Read the model definition and answer for the solid it produces. Units are mm, in the model's axes. A direction names the side the tool comes from. Round coordinates to 2 decimals unless told otherwise and drop trailing zeros. Write each loop counter-clockwise with the first axis right and the second up, starting at its lowest first coordinate (ties: lowest second). Pieces come first, ordered by that corner, then holes. Notation, with made-up numbers: (-9, 89) - (21, 89) arc R20 cw to (21, 111) - close; hole circle Ø9 at (-25.5, 72.25). An arc over 180 degrees is marked (long way). Answer as CSV lines item,"result". Start each with the question number.
1) Each of these flat-tipped pins is pushed along its axis until it touches: pin 1 (8 mm diameter, centred on x = 15.5, y = 5, fed in from +Z); pin 2 (8 mm diameter, centred on y = 12.5, z = 2.5, fed in from +X). Where does it stop, or does it pass through?
2) Find section D-D on z = 4.5. Determine the outline of the cut face in (x, y).
3) Find section A-A on x = 21.25. Determine the outline of the cut face in (y, z).
4) For a pull along Y with two mould halves and no side action, classify faces 3 (the flat face through (10, 0, 13)), 4 (the flat face through (10, 25.4, 13)), 5 (the flat face through (11, 23.812, 15)), 6 (the flat face through (1, 13, 0)) as +Y half, -Y half, draft (parallel to the pull), parting line (faces both ways), or undercut.
5) Find section C-C on y = 2.75. Determine the outline of the cut face in (x, z), then the cut area to 3 significant figures.
6) Which of the six approach directions +Z, -Z, +X, -X, +Y, -Y give full straight-line access (tool end or side, diameter ignored) to faces 1 (the flat face through (1.588, 13, 13)), 2 (the flat face through (1, 13, 25.4))?
7) Find section B-B on z = 16.75. Determine the outline of the cut face in (x, y).
8) Consider line 1 along Y through (x, z) = (4.75, 16.25); line 2 along Y through (x, z) = (0.8, 12.7); line 3 along X through (y, z) = (0.4, 12.7). Determine where each line is inside the solid, lowest interval first.
from build123d import *

# Parameters (mm, degrees)
EXTRUDE_THIN1_DEPTH = 25.4
SKETCH3_R           = 3.175
CUT_EXTRUDE1_DEPTH  = 44.097043475
FILLET1_R           = 12.7
SKETCH5_W           = 25.4
SKETCH5_H           = 1.5875
BOSS_EXTRUDE1_DEPTH = 25.4
SKETCH6_R           = 3.175
CUT_EXTRUDE3_DEPTH  = 25.4


with BuildPart() as part:
    # Sketch1 → Extrude-Thin1 (new body)
    with BuildSketch(Plane.XY):
        Polygon((0, 25.4), (0, 0), (25.4, 0), (25.4, 1.5875), (1.5875, 1.5875), (1.5875, 25.4), align=None)
    extrude(amount=EXTRUDE_THIN1_DEPTH)

    # Sketch3 → Cut-Extrude1 (cut, through all)
    with BuildSketch(Plane(origin=(1.5875, 0, 0), x_dir=(0, 0, -1), z_dir=(1, 0, 0))):
        with Locations((-12.7, 16.933333333)):
            Circle(SKETCH3_R)
        with Locations((-12.7, 8.466666667)):
            Circle(SKETCH3_R)
    extrude(amount=-CUT_EXTRUDE1_DEPTH, mode=Mode.SUBTRACT)

    # Fillet1
    fillet1_edges = [part.edges().sort_by_distance(p)[0] for p in [
        (25.4, 0.79375, 0),
        (25.4, 0.79375, 25.4),
    ]]
    fillet(fillet1_edges, radius=FILLET1_R - 0.0001)  # a hair under: the kernel refuses the full size

    # Sketch5 → Boss-Extrude1 (add)
    with BuildSketch(Plane.ZY):
        with Locations((12.7, 24.60625)):
            Rectangle(SKETCH5_W, SKETCH5_H)
    extrude(amount=-BOSS_EXTRUDE1_DEPTH)

    # Sketch6 → Cut-Extrude3 (cut)
    with BuildSketch(Plane(origin=(0, 25.4, 0), x_dir=(1, 0, 0), z_dir=(0, 1, 0))):
        with Locations(Location((13.49375, -12.7, 0), (0, 0, 270))):
            Circle(SKETCH6_R)
        with BuildLine():
            Line((25.4, -25.4), (25.4, -12.7))
            ThreePointArc((25.4, -12.7), (21.680256104, -21.680256138), (12.699999951, -25.4))
            Line((12.699999951, -25.4), (25.4, -25.4))
        make_face()
        with BuildLine():
            ThreePointArc((12.7, 0), (21.680256121, -3.719743879), (25.4, -12.7))
            Line((25.4, -12.7), (25.4, 0))
            Line((25.4, 0), (12.7, 0))
        make_face()
    extrude(amount=-CUT_EXTRUDE3_DEPTH, mode=Mode.SUBTRACT)


solid = part.part
Check values:
1,pin 1,"stops at z = 25.38"
1,pin 2,"stops at x = 1.59"
2,outline,"(0, 0) - (22.4, 0) - (22.4, 1.59) - (1.59, 1.59) - (1.59, 23.81) - (22.4, 23.81) - (22.4, 25.4) - (0, 25.4) - close"
3,outline,"(0, 3.31) - (1.59, 3.31) - (1.59, 22.09) - (0, 22.09) - close; (23.81, 3.31) - (25.4, 3.31) - (25.4, 22.09) - (23.81, 22.09) - close"
4,face 3,"-Y half"
4,face 4,"+Y half"
4,face 5,"undercut"
4,face 6,"draft"
5,outline,"(0, 0) - (1.59, 0) - (1.59, 25.4) - (0, 25.4) - close"
5,area,"40.3 mm^2"
6,face 1,"+Z, -Z, +X"
6,face 2,"+Z, +X, -X, +Y, -Y"
7,outline,"(0, 0) - (24.74, 0) - (24.74, 1.59) - (1.59, 1.59) - (1.59, 23.81) - (24.74, 23.81) - (24.74, 25.4) - (0, 25.4) - close"
8,line 1,"y = 0 to 1.59, 23.81 to 25.4"
8,line 2,"y = 0 to 5.29, 11.64 to 13.76, 20.11 to 25.4"
8,line 3,"x = 0 to 10.32, 16.67 to 25.4"
